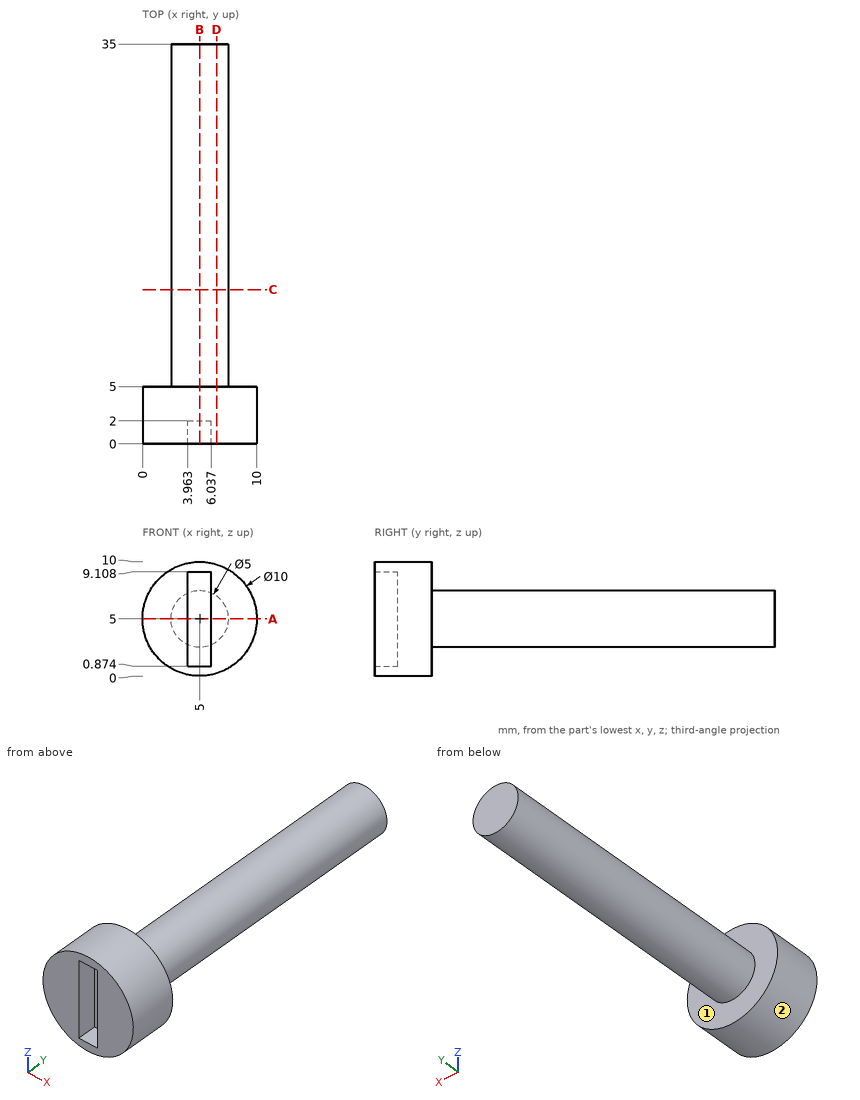
Could you check a few things on this drawing? It's one solid part, dimensions in mm from its lowest x, y, z. A direction names the side the tool comes from. Coordinates: 2 decimals unless noted, no trailing zeros. Write each loop counter-clockwise with the first axis right and the second up, starting at its lowest first coordinate (ties: lowest second). Pieces come first, ordered by that corner, then holes.
Q1. Imagine slicing it at D-D, the plane x = 6.5. List the corners of the cut face in (y, z) for me.
Results found:
outline: (0, 0.23) - (5, 0.23) - (5, 3) - (35, 3) - (35, 7) - (5, 7) - (5, 9.77) - (0, 9.77) - close
Q2. Please list where these lines run through material, in increasing order: L1, parallel to Y at x = 7.25, z = 8.25; L2, parallel to X at y = 15.5, z = 5.5; L3, parallel to Z at x = 3.25, y = 15 (1 decimal).
Results found:
L1: y = 0 to 5
L2: x = 2.55 to 7.45
L3: z = 3.2 to 6.8
Q3. Imagine slicing it at A-A, the plane z = 5. List the corners of the cut face in (x, y) for me.
Results found:
outline: (0, 0) - (3.96, 0) - (3.96, 2) - (6.04, 2) - (6.04, 0) - (10, 0) - (10, 5) - (7.5, 5) - (7.5, 35) - (2.5, 35) - (2.5, 5) - (0, 5) - close
Q4. Imagine slicing it at B-B, the plane x = 5. List the corners of the cut face in (y, z) for me.
Results found:
outline: (0, 0) - (5, 0) - (5, 2.5) - (35, 2.5) - (35, 7.5) - (5, 7.5) - (5, 10) - (0, 10) - (0, 9.11) - (2, 9.11) - (2, 0.87) - (0, 0.87) - close
Q5. Which directions (+Z, -Z, +X, -X, +Y, -Y) give clear straight access to the entire face, cutting with the end or side of a thin tool? Please do the marked faces 1 and 2.
Results found:
face 1: +Y
face 2: +Y, -Y
Q6. Imagine slicing it at C-C, the plane y = 13.5. List the corners of the cut face in (x, z) for me.
Results found:
outline: circle Ø5 at (5, 5)
Q7. For P1, Ø1.7, axis at x = 5, z = 3.5, coming from the -Y side; P2, Ø0.6, axis at y = 0.5, z = 3.5, coming from the -X side; P3, Ø1, axis at x = 8.5, z = 7.5, coming from the +Y side, each with a flat end and sliding along its axis, tell me the tip position at first contact or that it passes through.
Results found:
P1: stops at y = 2
P2: stops at x = 0.15
P3: stops at y = 5
